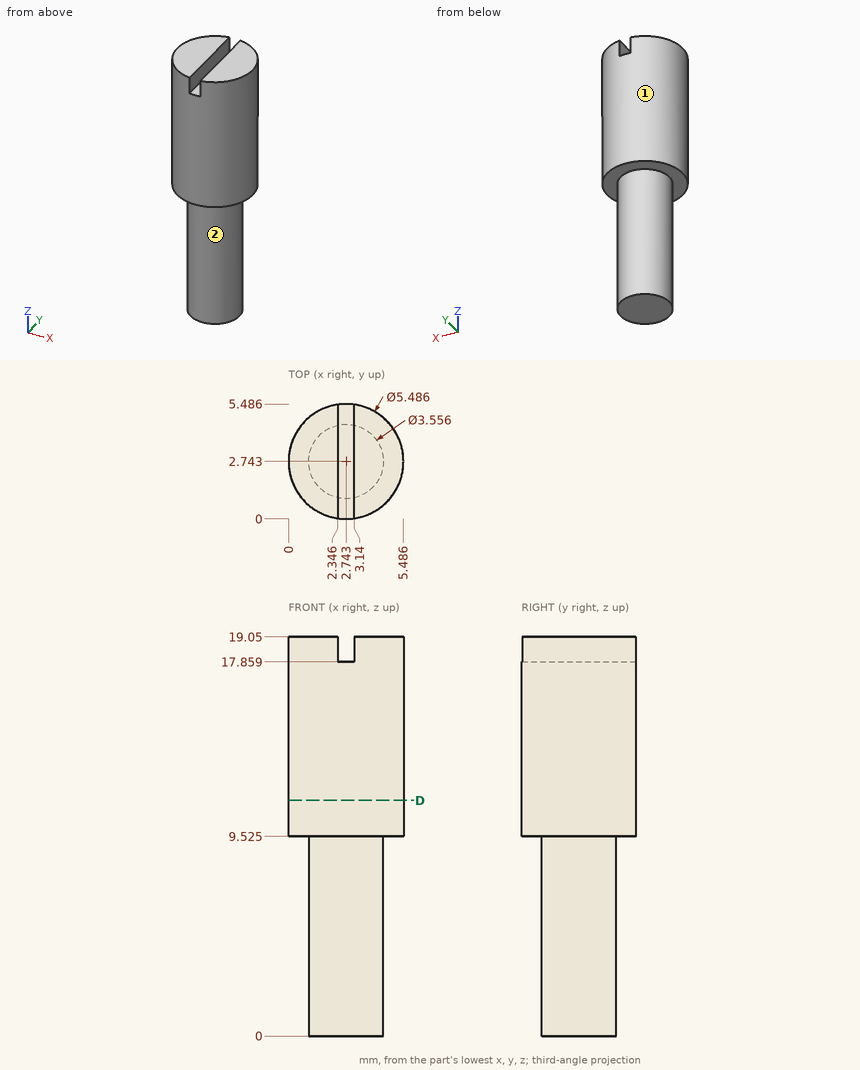
Input: dimensioned drawing with shaded views. Units: mm. Origin: part minimum x, y, z. A direction names the side the tool comes from. Round coordinates to 2 decimals unless told otherwise and drop trailing zeros. Loops run counter-clockwise (first coordinate to the right, second up) from the corner with the lowest first, then second, coordinate; pieces in that order, holes last.
1) Section query D-D on z = 11.25. Return the cut outline in (x, y).
Ans:
outline: circle Ø5.49 at (2.74, 2.74)
2) Set-up query: the marked faces 1 and 2. Return all of +Z, -Z, +X, -X, +Y, -Y with unobstructed straight access to the full face (end or side cutting, diameter ignored); none if empty.
Ans:
face 1: +Z, -Z
face 2: -Z
3) Pin query (flat end, axial travel): pin 1 (1 mm diameter, centred on x = 4.5, z = 13.5, fed in from -Y) (1 decimal); pin 2 (1.3 mm diameter, centred on y = 2.5, z = 18.5, fed in from +X); pin 3 (1.5 mm diameter, centred on y = 4, z = 7, fed in from +X); pin 4 (0.6 mm diameter, centred on y = 2, z = 18.5, fed in from -X). Return the tip coordinate at first contact, or that it passes through.
Ans:
pin 1: stops at y = 0.3
pin 2: stops at x = 5.49
pin 3: stops at x = 4.45
pin 4: stops at x = 0.04
4) Material intervals for line 1 (Z direction, x = 2.55, y = 4.15); line 2 (X direction, y = 3.15, z = 11) (1 decimal); line 3 (X direction, y = 4.2, z = 16.25), sorted ascending.
Ans:
line 1: z = 0 to 17.86
line 2: x = 0 to 5.5
line 3: x = 0.42 to 5.07
